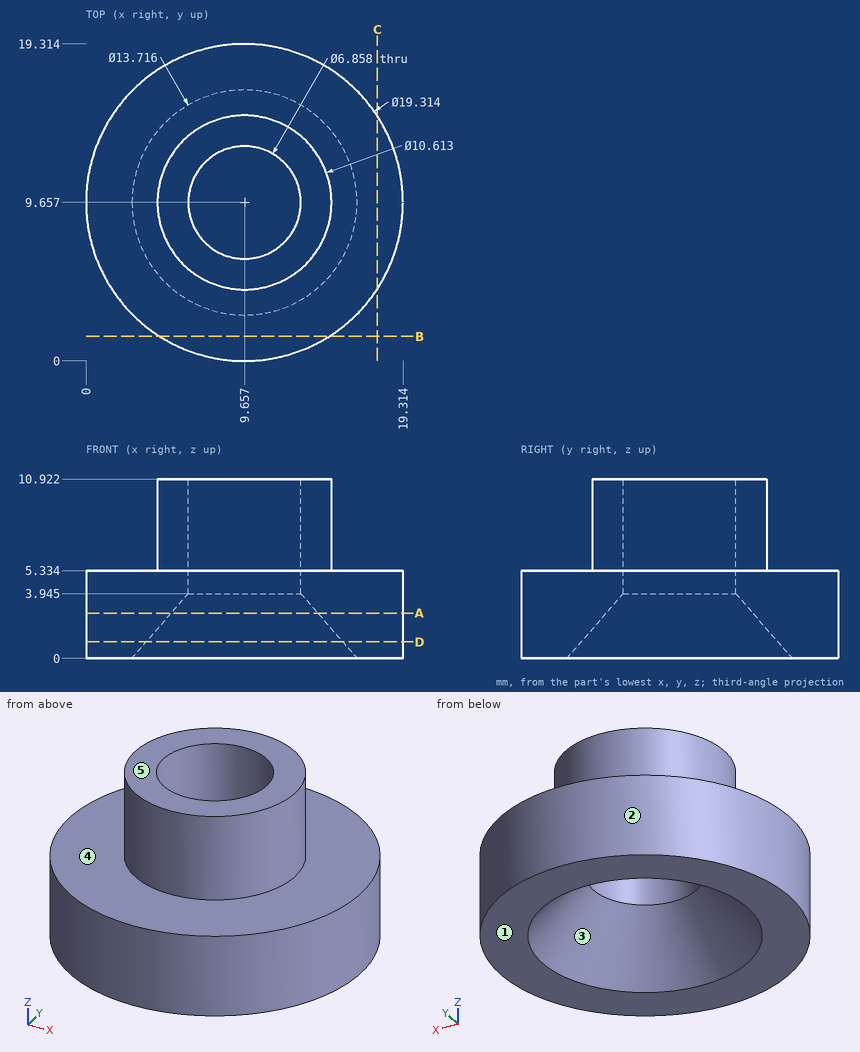
Source: three-view drawing plus pictorial views. Frame: mm from the lowest corner of the part. A direction names the side the tool comes from. Coordinates: 2 decimals unless noted, no trailing zeros. Order: outer loops, then holes, each group sorted by start corner. A loop starts at its lowest first (then second) coordinate and runs counter-clockwise, first axis right, second up. Notation, with made-up numbers: M 0.5,5 L 18.5,5 A33 ccw 18.5,44 Z; hole C -18.5,71 d5. An arc over 180 degrees is marked long. One line per question, with ' | ' between items.
Item 1: Section C-C (x = 17.75). Output: boundary loops of the cut face in (y, z) (1 decimal), then the cut area to 3 significant figures.
Geometry results:
outline: M 4.4,0 L 14.9,0 L 14.9,5.3 L 4.4,5.3 Z | area: 56.2 mm^2
Item 2: Section B-B (y = 1.5). Output: boundary loops of the cut face in (x, z).
Geometry results:
outline: M 4.49,0 L 14.83,0 L 14.83,5.33 L 4.49,5.33 Z
Item 3: Draft query along Y for the marked faces 1, 2 and 3. Return one class per face: released by +Y, released by -Y, zero draft, split by the parting line, or undercut.
Geometry results:
face 1: zero draft | face 2: split by the parting line | face 3: undercut
Item 4: Section A-A (z = 2.75). Output: boundary loops of the cut face in (x, y) (1 decimal), then the cut area to 3 significant figures.
Geometry results:
outline: C 9.7,9.7 d19.3; hole C 9.7,9.7 d8.9 | area: 230 mm^2
Item 5: Ray query, line 1 along Y through (x, z) = (9.5, 6); line 2 along X through (y, z) = (12, 1.5) (1 decimal); line 3 along Y through (x, z) = (8.25, 9.5) (1 decimal). Return the intervals inside material, ascending.
Geometry results:
line 1: y = 4.35 to 6.23, 13.08 to 14.96 | line 2: x = 0.3 to 4.6, 14.7 to 19 | line 3: y = 4.5 to 6.5, 12.8 to 14.8
Item 6: Pin query (flat end, axial travel): pin 1 (1 mm diameter, centred on x = 5.5, z = 7.5, fed in from +Y); pin 2 (1.5 mm diameter, centred on x = 7.5, z = 7.5, fed in from -Y); pin 3 (6 mm diameter, centred on x = 6, z = 5.5, fed in from +Y). Return the tip coordinate at first contact, or that it passes through.
Geometry results:
pin 1: stops at y = 13.5 | pin 2: stops at y = 4.54 | pin 3: stops at y = 19.29
Item 7: Reachability of the marked faces 4 and 5 from +Z, -Z, +X, -X, +Y, -Y: full face, straight path, thin tool, end or side. Return the list, or none.
Geometry results:
face 4: +Z | face 5: +Z, +X, -X, +Y, -Y
Item 8: Section D-D (z = 1). Output: boundary loops of the cut face in (x, y).
Geometry results:
outline: C 9.66,9.66 d19.31; hole C 9.66,9.66 d11.98
